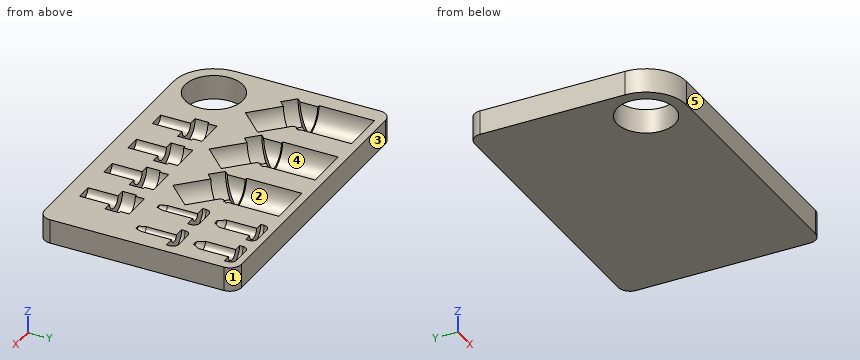
```python
from build123d import *

# Parameters (mm, degrees)
F0_R      = 12.5
F1_DEPTH  = 10.5
F10_START = -9.5
F9_R      = 12.5
F10_DEPTH = 1


with BuildPart() as f1:
    # F0 (on Top) → F1 (new body)
    with BuildSketch(Plane.XY):
        with BuildLine():
            ThreePointArc((0, 17.5), (5.1256313292, 5.1256313292), (17.5, 0))
            Line((17.5, 0), (124, 0))
            ThreePointArc((124, 0), (127.5355339059, 1.4644660941), (129, 5))
            Line((129, 5), (129, 80))
            ThreePointArc((129, 80), (127.5355339059, 83.5355339059), (124, 85))
            Line((124, 85), (5, 85))
            ThreePointArc((5, 85), (1.4644660941, 83.5355339059), (0, 80))
            Line((0, 80), (0, 17.5))
        make_face()
        with Locations((17.5, 17.5)):
            Circle(F0_R, mode=Mode.SUBTRACT)
    extrude(amount=F1_DEPTH)

    # F2 (on face) → F3 (revolve, cut)
    with BuildSketch(Plane.XY.offset(10.5)):
        Polygon((14.3187418757, 55.9630800428), (16.818928037, 53.5137803146), (16.818928037, 81.5137803146), (7.318928037, 81.5137803146), (7.318928037, 57.5137803146), (8.318928037, 57.5137803146), (8.318928037, 53.1566108629), (8.318928037, 49.8386146061), align=None)
        Polygon((8.318928037, 49.5137803146), (16.818928037, 53.5137803146), (14.3187418757, 55.9630800428), (8.318928037, 49.8386146061), align=None)
    revolve(axis=Axis((16.818928037, 67.5137803146, 10.5), (0, 1, 0)), mode=Mode.SUBTRACT)

    # F2 (on face) → F4 (revolve, cut)
    with BuildSketch(Plane.XY.offset(10.5)):
        Polygon((44.3187418757, 55.9630800428), (46.818928037, 53.5137803146), (46.818928037, 81.5137803146), (37.318928037, 81.5137803146), (37.318928037, 57.5137803146), (38.318928037, 57.5137803146), (38.318928037, 49.8386146061), align=None)
    revolve(axis=Axis((46.818928037, 67.5137803146, 10.5), (0, 1, 0)), mode=Mode.SUBTRACT)

    # F2 (on face) → F5 (revolve, cut)
    with BuildSketch(Plane.XY.offset(10.5)):
        Polygon((74.3187418757, 55.9630800428), (76.818928037, 53.5137803146), (76.818928037, 81.5137803146), (67.318928037, 81.5137803146), (67.318928037, 57.5137803146), (68.318928037, 57.5137803146), (68.318928037, 49.8386146061), align=None)
    revolve(axis=Axis((76.818928037, 67.5137803146, 10.5), (0, 1, 0)), mode=Mode.SUBTRACT)

    # F2 (on face) → F6 (revolve, cut)
    with BuildSketch(Plane.XY.offset(10.5)):
        Polygon((14.0706147806, 45.7069388121), (25, 35), (30.2484994177, 40.3575417742), (16.818928037, 53.5137803146), (8.318928037, 49.5137803146), (8.318928037, 49.8386146061), (6.6209427297, 48.1053521073), (11.6213150523, 43.2067526508), align=None)
        Polygon((8.318928037, 49.5137803146), (16.818928037, 53.5137803146), (14.3187418757, 55.9630800428), (8.318928037, 49.8386146061), align=None)
    revolve(axis=Axis((22.2836206467, 48.1603109085, 10.5), (0.7143389032, -0.6997999224, 0)), mode=Mode.SUBTRACT)

    # F2 (on face) → F7 (revolve, cut)
    with BuildSketch(Plane.XY.offset(10.5)):
        Polygon((60.2484994177, 40.3575417742), (46.818928037, 53.5137803146), (38.318928037, 49.5137803146), (38.318928037, 49.8386146061), (36.6209427297, 48.1053521073), (41.6213150523, 43.2067526508), (44.0706147806, 45.7069388121), (55, 35), align=None)
        Polygon((38.318928037, 49.5137803146), (46.818928037, 53.5137803146), (44.3187418757, 55.9630800428), (38.318928037, 49.8386146061), align=None)
    revolve(axis=Axis((53.5337137273, 46.9356610444, 10.5), (0.7143389032, -0.6997999224, 0)), mode=Mode.SUBTRACT)

    # F2 (on face) → F8 (revolve, cut)
    with BuildSketch(Plane.XY.offset(10.5)):
        Polygon((90.2484994177, 40.3575417742), (76.818928037, 53.5137803146), (68.318928037, 49.5137803146), (68.318928037, 49.8386146061), (66.6209427297, 48.1053521073), (71.6213150523, 43.2067526508), (74.0706147806, 45.7069388121), (85, 35), align=None)
        Polygon((68.318928037, 49.5137803146), (76.818928037, 53.5137803146), (74.3187418757, 55.9630800428), (68.318928037, 49.8386146061), align=None)
    revolve(axis=Axis((83.5337137273, 46.9356610444, 10.5), (0.7143389032, -0.6997999224, 0)), mode=Mode.SUBTRACT)

    # F9 (on face) → F10 (join)
    with BuildSketch(Plane.XY.offset(10.5).offset(F10_START)):
        with BuildLine():
            ThreePointArc((129, 80), (127.5355339059, 83.5355339059), (124, 85))
            Line((124, 85), (5, 85))
            ThreePointArc((5, 85), (1.4644660941, 83.5355339059), (0, 80))
            Line((0, 80), (0, 17.5))
            ThreePointArc((0, 17.5), (5.1256313292, 5.1256313292), (17.5, 0))
            Line((17.5, 0), (124, 0))
            ThreePointArc((124, 0), (127.5355339059, 1.4644660941), (129, 5))
            Line((129, 5), (129, 80))
        make_face()
        with Locations((17.5, 17.5)):
            Circle(F9_R, mode=Mode.SUBTRACT)
    extrude(amount=-F10_DEPTH)

    # F11 (on face) → F12 (revolve, cut)
    with BuildSketch(Plane.XY.offset(10.5)):
        with BuildLine():
            Line((104.75, 82), (101, 82))
            Line((101, 82), (101, 78))
            Line((101, 78), (101, 72))
            Line((101, 72), (101, 62))
            Line((101, 62), (102, 62))
            Line((102, 62), (104, 65))
            Line((104, 65), (104, 78))
            Line((104, 78), (107.25, 78))
            Line((107.25, 78), (107.25, 79.5))
            ThreePointArc((107.25, 79.5), (106.517766953, 81.267766953), (104.75, 82))
        make_face()
        with BuildLine():
            Line((104.75, 57), (101, 57))
            Line((101, 57), (101, 53))
            Line((101, 53), (101, 37))
            Line((101, 37), (102, 37))
            Line((102, 37), (103, 40))
            Line((103, 40), (103, 53))
            Line((103, 53), (107.25, 53))
            Line((107.25, 53), (107.25, 54.5))
            ThreePointArc((107.25, 54.5), (106.517766953, 56.267766953), (104.75, 57))
        make_face()
    revolve(axis=Axis((101, 45, 10.5), (0, -1, 0)), mode=Mode.SUBTRACT)

    # F11 (on face) → F13 (revolve, cut)
    with BuildSketch(Plane.XY.offset(10.5)):
        Polygon((121.5, 78), (118.5, 78), (118.5, 62), (119.5, 62), (121.5, 65), align=None)
        with BuildLine():
            Line((122.25, 82), (118.5, 82))
            Line((118.5, 82), (118.5, 78))
            Line((118.5, 78), (121.5, 78))
            Line((121.5, 78), (124.75, 78))
            Line((124.75, 78), (124.75, 79.5))
            ThreePointArc((124.75, 79.5), (124.017766953, 81.267766953), (122.25, 82))
        make_face()
        with BuildLine():
            Line((122.25, 57), (118.5, 57))
            Line((118.5, 57), (118.5, 53))
            Line((118.5, 53), (118.5, 37))
            Line((118.5, 37), (119.5, 37))
            Line((119.5, 37), (120.5, 40))
            Line((120.5, 40), (120.5, 53))
            Line((120.5, 53), (124.75, 53))
            Line((124.75, 53), (124.75, 54.5))
            ThreePointArc((124.75, 54.5), (124.017766953, 56.267766953), (122.25, 57))
        make_face()
    revolve(axis=Axis((118.5, 45, 10.5), (0, -1, 0)), mode=Mode.SUBTRACT)

    # F14 (on face) → F15 (revolve, cut)
    with BuildSketch(Plane.XY.offset(10.5)):
        Polygon((51.25, 30), (45, 30), (45, 26), (45, 20), (45, 17.5), (45, 7), (48.5, 7), (48.5, 20), (52.25, 20), (52.25, 26), (51.25, 26), align=None)
    revolve(axis=Axis((45, 13.5, 10.5), (0, -1, 0)), mode=Mode.SUBTRACT)

    # F14 (on face) → F16 (revolve, cut)
    with BuildSketch(Plane.XY.offset(10.5)):
        Polygon((71.25, 30), (65, 30), (65, 26), (65, 20), (65, 7), (68.5, 7), (68.5, 20), (72.25, 20), (72.25, 26), (71.25, 26), align=None)
    revolve(axis=Axis((65, 13.5, 10.5), (0, -1, 0)), mode=Mode.SUBTRACT)

    # F14 (on face) → F17 (revolve, cut)
    with BuildSketch(Plane.XY.offset(10.5)):
        Polygon((91.25, 30), (85, 30), (85, 26), (85, 20), (85, 7), (88.5, 7), (88.5, 20), (92.25, 20), (92.25, 26), (91.25, 26), align=None)
    revolve(axis=Axis((85, 13.5, 10.5), (0, -1, 0)), mode=Mode.SUBTRACT)

    # F14 (on face) → F18 (revolve, cut)
    with BuildSketch(Plane.XY.offset(10.5)):
        Polygon((111.25, 30), (105, 30), (105, 26), (105, 20), (105, 7), (108.5, 7), (108.5, 20), (112.25, 20), (112.25, 26), (111.25, 26), align=None)
    revolve(axis=Axis((105, 13.5, 10.5), (0, -1, 0)), mode=Mode.SUBTRACT)


solid = f1.part
```
CAD build for the part. Positions are in the model's coordinates, mm. Face numbers are marked on the shaded views. A direction names the side the tool comes from. Round coordinates to 2 decimals unless told otherwise and drop trailing zeros. Order: outer loops, then holes, each group sorted by start corner. A loop starts at its lowest first (then second) coordinate and runs counter-clockwise, first axis right, second up.
Q1. Slice it at A-A (y = 27.5). Write the cut outline in (x, z).
Q2. Two-plate mould, pull along Y, no slides. Class the marked faces 3, 4 and 5: pulls with the +Y half, pulls with the -Y half, needs draft (parallel to the pull), parting line crosses it, or undercut.
Q3. Drop flat-ended pins along their axis: pin 1 (14 mm diameter, centred on x = 17, y = 56, fed in from +Z); pin 2 (1.5 mm diameter, centred on x = 54.5, y = 71.5, fed in from +Z). Give the stop position or say it passes through.
Q4. Slice it at B-B (y = 68.5). Write the cut outline in (x, z), and give its area (3 significant figures).
Q5. Which spindle directions (+Z, -Z, +X, -X, +Y, -Y) get a long thin tool onto all of the face, cutting with end or side? Do the marked faces 1 and 2. Say none if no direction does.
Q6. Wall check: L1, parallel to Y at x = 17.5, z = 7.5; L2, parallel to Y at x = 56, z = 7.25; L3, parallel to X at y = 15, z = 9. Give the ranges that are in metal, low to high.
Results below:
1. outline: (0, 0) - (10, 0) - (10, 10.5) - (0, 10.5) - close; (25, 0) - (129, 0) - (129, 10.5) - (111.25, 10.5) arc R6.25 cw to (98.75, 10.5) - (91.25, 10.5) arc R6.25 cw to (78.75, 10.5) - (71.25, 10.5) arc R6.25 cw to (58.75, 10.5) - (51.25, 10.5) arc R6.25 cw to (38.75, 10.5) - (25, 10.5) - close
2. face 3: pulls with the +Y half
2. face 4: undercut
2. face 5: pulls with the -Y half
3. pin 1: stops at z = 5.95
3. pin 2: stops at z = 6.12
4. outline: (0, 0) - (129, 0) - (129, 10.5) - (121.5, 10.5) arc R3 cw to (115.5, 10.5) - (104, 10.5) arc R3 cw to (98, 10.5) - (86.32, 10.5) arc R9.5 cw to (67.32, 10.5) - (56.32, 10.5) arc R9.5 cw to (37.32, 10.5) - (26.32, 10.5) arc R9.5 cw to (7.32, 10.5) - (0, 10.5) - close
4. area: 901 mm2
5. face 1: +Z, -Z, +X, +Y
5. face 2: +Z
6. L1: y = 0 to 5, 30 to 43.22, 81.51 to 85
6. L2: y = 0 to 36.02, 53.98 to 57.88, 59.23 to 85
6. L3: x = 0.18 to 5.25, 29.75 to 41.84, 48.16 to 61.84, 68.16 to 81.84, 88.16 to 101.84, 108.16 to 129
